Check sheet for the modelled part. Datum: model origin and axes. Units: mm. Face numbers are marked on the shaded views. A direction names the side the tool comes from. Coordinates: 2 decimals unless noted, no trailing zeros. Order: outer loops, then holes, each group sorted by start corner. A loop starts at its lowest first (then second) coordinate and runs counter-clockwise, first axis right, second up.
1. Thickness scan on line 1 (Y direction, x = 0, z = 6.25); line 2 (Y direction, x = 0, z = 19.75); line 3 (Y direction, x = -9.5, z = 9). Record the ranges inside material, lowest first.
2. Cross-section at A-A (y = -8). Enter the section's corners in (x, z).
3. Cross-section at B-B (x = 9.5). Enter the section's corners in (y, z), then the cut area to 3 significant figures.
4. Draft check along Y on the marked faces 3, 4 and 5. Enter one of: released by +Y, released by -Y, zero draft, split by the parting line, or undercut.
5. Gauge pin test, flat ends, axial feed: pin 1 Ø4 at (x, y) = (0, 9.5) entering from -Z; pin 2 Ø2 at (y, z) = (-0.5, 20) entering from +X; pin 3 Ø12 at (x, y) = (-7.5, -11.5) entering from +Z; pin 4 Ø4 at (x, y) = (0, 0) entering from +Z. Record the tip position at first contact, or that the pin passes through.
6. Cross-section at D-D (z = 12.5). Enter the section's corners in (x, y).
7. Cross-section at C-C (z = 6.75). Enter the section's corners in (x, y).
8. Set-up check for the marked faces 1 and 2: record each of +Z, -Z, +X, -X, +Y, -Y from which the full face is reachable in a straight line by a thin tool's end or side.
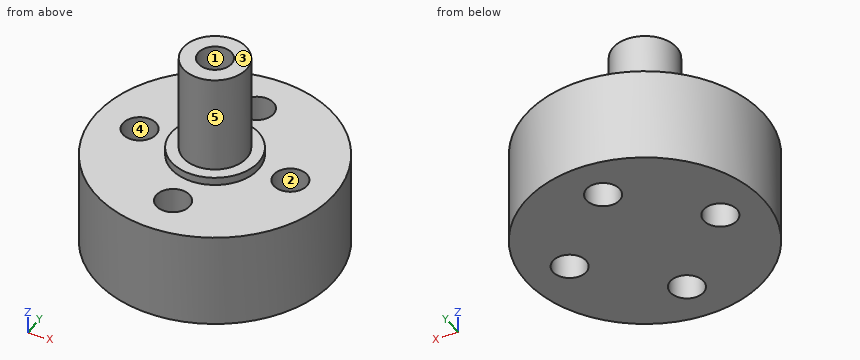
```python
from build123d import *

# Parameters (mm, degrees)
SKETCH_1_R      = 15
EXTRUDE_1_DEPTH = 12
SKETCH_2_R      = 5.5
EXTRUDE_2_DEPTH = 1
SKETCH_3_R      = 4
EXTRUDE_3_DEPTH = 12.4
M5X0_81_D       = 4.2
M5X0_82_D       = 4.2
M5X0_82_DEPTH   = 14
M5X0_82_TIP     = 1.2618073


with BuildPart() as part:
    # Эскиз1 → Бобышка-Вытянуть1 (new body)
    with BuildSketch(Plane.XY):
        Circle(SKETCH_1_R)
    extrude(amount=EXTRUDE_1_DEPTH)

    # Эскиз2 → Бобышка-Вытянуть2 (add)
    with BuildSketch(Plane.XY.offset(12)):
        Circle(SKETCH_2_R)
    extrude(amount=EXTRUDE_2_DEPTH)

    # Эскиз3 → Бобышка-Вытянуть3 (add)
    with BuildSketch(Plane.XY.offset(13)):
        with Locations(Location((0, 0, 0), (0, 0, 180))):
            Circle(SKETCH_3_R)
    extrude(amount=EXTRUDE_3_DEPTH)

    # Отверстие обработанное метчиком M5x0.81 (through all)
    with Locations(Plane(origin=(0, 0, 0), x_dir=(-1, 0, 0), z_dir=(0, 0, -1))):
        with Locations((0, 9.5), (9.5, 0), (-9.5, 0), (0, -9.5)):
            Hole(M5X0_81_D / 2)

    # Отверстие обработанное метчиком M5x0.82
    with Locations(Plane.XY.offset(25.4)):
        with Locations((0, 0)):
            Hole(M5X0_82_D / 2, depth=M5X0_82_DEPTH)
            with Locations((0, 0, -(M5X0_82_DEPTH + M5X0_82_TIP / 2))):  # 118° drill point
                Cone(0, M5X0_82_D / 2, M5X0_82_TIP, mode=Mode.SUBTRACT)


solid = part.part
```
Data:
1. line 1: y = -15 to -11.6, -7.4 to 7.4, 11.6 to 15
1. line 2: y = -4 to -2.1, 2.1 to 4
1. line 3: y = -11.61 to -2.1, 2.1 to 11.61
2. outline: (-12.69, 0) - (-1.47, 0) - (-1.47, 12) - (-12.69, 12) - close; (1.47, 0) - (12.69, 0) - (12.69, 12) - (1.47, 12) - close
3. outline: (-11.61, 0) - (-2.1, 0) - (-2.1, 12) - (-11.61, 12) - close; (2.1, 0) - (11.61, 0) - (11.61, 12) - (2.1, 12) - close
3. area: 228 mm2
4. face 3: zero draft
4. face 4: undercut
4. face 5: split by the parting line
5. pin 1: passes through
5. pin 2: stops at x = 4
5. pin 3: stops at z = 12
5. pin 4: stops at z = 11.34
6. outline: circle Ø11 at (0, 0); hole circle Ø4.2 at (0, 0)
7. outline: circle Ø30 at (0, 0); hole circle Ø4.2 at (-9.5, 0); hole circle Ø4.2 at (0, -9.5); hole circle Ø4.2 at (0, 9.5); hole circle Ø4.2 at (9.5, 0)
8. face 1: +Z
8. face 2: +Z, -Z
